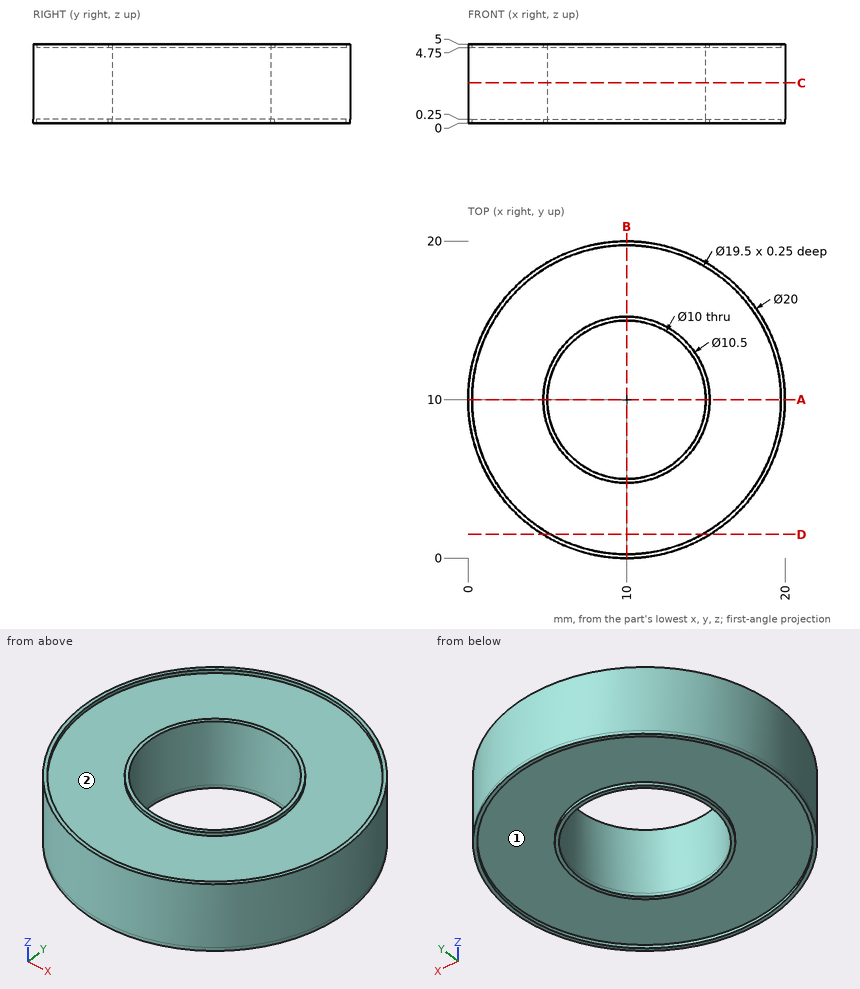
Job drawing, mm, ordinate dimensions from the low corner. One solid piece. A direction names the side the tool comes from. Give positions to 0.01 mm unless a question says otherwise; leave off trailing zeros. Write each loop counter-clockwise with the first axis right and the second up, starting at its lowest first coordinate (ties: lowest second). Pieces come first, ordered by that corner, then holes. Notation, with made-up numbers: (-34, 67) - (-5, 67) arc R28 ccw to (-5, 95) - close; hole circle Ø9 at (37, 72). An arc over 180 degrees is marked (long way). Use one line per item in the form item = value. Start each with the question number.
1. Band-saw the part on D-D on y = 1.5. Write the cut outline in (x, z).
2. Band-saw the part on A-A on y = 10. Write the cut outline in (x, z), plus the area to 3 significant figures.
3. Drop flat-ended pins along their axis: pin 1 Ø4 at (x, y) = (5.5, 4) entering from -Z; pin 2 Ø6 at (x, y) = (10, 10) entering from +Z. Give the stop position or say it passes through.
4. 3-axis set-ups, long thin cutter, end or side, ignore diameter. For the marked faces 1 and 2: which of +Z, -Z, +X, -X, +Y, -Y reach the whole face in a straight line?
5. Band-saw the part on C-C on z = 2.55. Write the cut outline in (x, y), plus the area to 3 significant figures.
6. Probe line 1 (Y direction, x = 10, z = 4.9); line 2 (X direction, y = 10, z = 2.2); line 3 (Z direction, x = 11.75, y = 18). List the from-to ranges inside material, lowest first. Write a range as [from, to].
Conclusion:
q1.outline = (4.73, 0) - (5.22, 0) - (5.22, 0.25) - (14.78, 0.25) - (14.78, 0) - (15.27, 0) - (15.27, 5) - (14.78, 5) - (14.78, 4.75) - (5.22, 4.75) - (5.22, 5) - (4.73, 5) - close
q2.outline = (0, 0) - (0.25, 0) - (0.25, 0.25) - (4.75, 0.25) - (4.75, 0) - (5, 0) - (5, 5) - (4.75, 5) - (4.75, 4.75) - (0.25, 4.75) - (0.25, 5) - (0, 5) - close; (15, 0) - (15.25, 0) - (15.25, 0.25) - (19.75, 0.25) - (19.75, 0) - (20, 0) - (20, 5) - (19.75, 5) - (19.75, 4.75) - (15.25, 4.75) - (15.25, 5) - (15, 5) - close
q2.area = 45.5 mm²
q3.pin_1 = 0.25
q3.pin_2 = through
q4.face_1 = -Z
q4.face_2 = +Z
q5.outline = circle Ø20 at (10, 10); hole circle Ø10 at (10, 10)
q5.area = 236 mm²
q6.line_1 = [0, 0.25], [4.75, 5], [15, 15.25], [19.75, 20]
q6.line_2 = [0, 5], [15, 20]
q6.line_3 = [0.25, 4.75]
